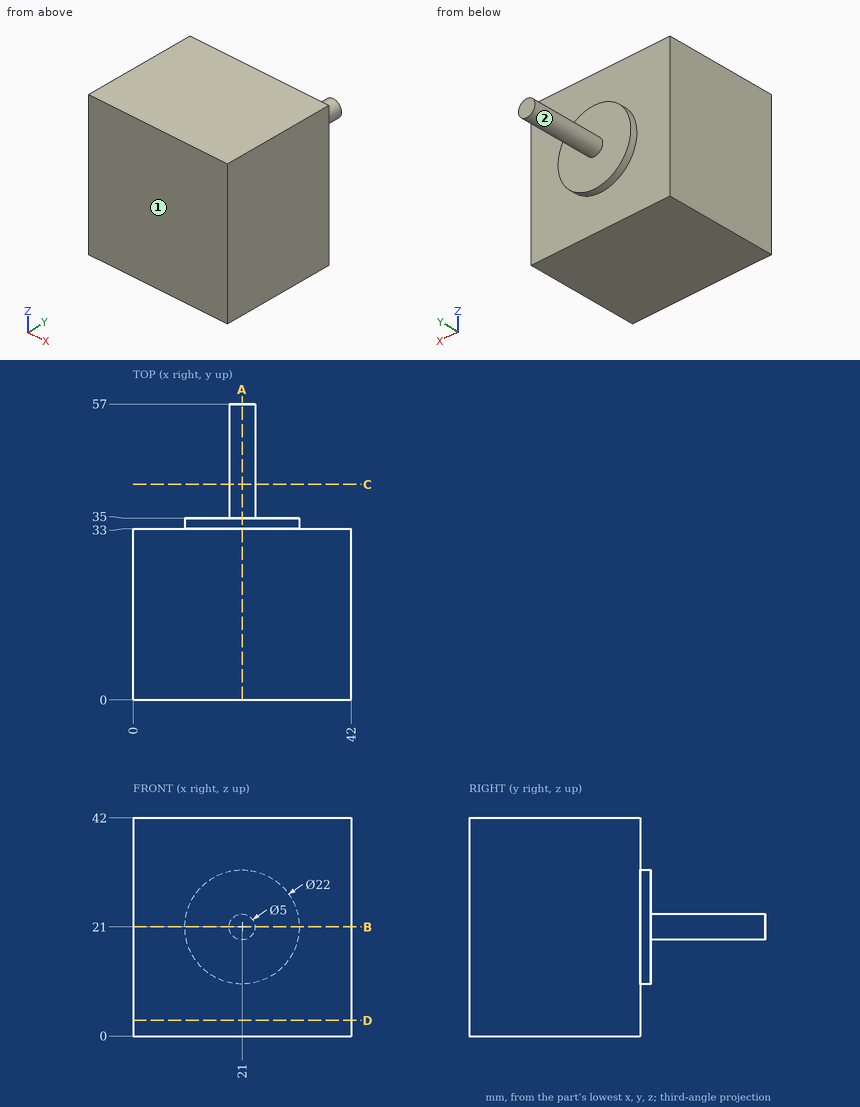
The figure shows three views and two pictorial views of one solid part (mm, origin at its lowest corner). Answer the questions. A direction names the side the tool comes from. Give positions to 0.01 mm unless a question says otherwise; leave off trailing zeros. Loops run counter-clockwise (first coordinate to the right, second up) from the corner with the lowest first, then second, coordinate; pieces in that order, holes last. Notation, with made-up numbers: (-19, 46) - (-3, 46) arc R32 cw to (-3, 76) - close; hole circle Ø4 at (-33, 83). An arc over 180 degrees is marked (long way). Use one line per item in the form item = value.
1. Find the intervals of material crossed by line 1 along Y through (x, z) = (21, 6); line 2 along Y through (x, z) = (22.5, 27); line 3 along X through (y, z) = (42, 19.5), in increasing order. Write a range as [from, to].
Calculated:
line_1 = [0, 33]
line_2 = [0, 35]
line_3 = [19, 23]
2. Section D-D on z = 3 is taken. Give the vertices of the cut face in (x, y).
Calculated:
outline = (0, 0) - (42, 0) - (42, 33) - (0, 33) - close
3. Section A-A on x = 21 is taken. Give the vertices of the cut face in (y, z).
Calculated:
outline = (0, 0) - (33, 0) - (33, 10) - (35, 10) - (35, 18.5) - (57, 18.5) - (57, 23.5) - (35, 23.5) - (35, 32) - (33, 32) - (33, 42) - (0, 42) - close
4. Section B-B on z = 21 is taken. Give the vertices of the cut face in (x, y), then the cut area to 3 significant figures.
Calculated:
outline = (0, 0) - (42, 0) - (42, 33) - (32, 33) - (32, 35) - (23.5, 35) - (23.5, 57) - (18.5, 57) - (18.5, 35) - (10, 35) - (10, 33) - (0, 33) - close
area = 1,540 mm^2
5. Section C-C on y = 41.5 is taken. Give the vertices of the cut face in (x, z), then the cut area to 3 significant figures.
Calculated:
outline = circle Ø5 at (21, 21)
area = 19.6 mm^2
6. Which of the six approach directions +Z, -Z, +X, -X, +Y, -Y give full straight-line access (tool end or side, diameter ignored) to the marked faces 1 and 2?
Calculated:
face_1 = +Z, -Z, +X, -X, -Y
face_2 = +Y
7. Given pin 1 Ø3 at (x, z) = (12.5, 25) entering from +Y; pin 2 Ø6 at (y, z) = (39.5, 19.5) entering from -X; pin 3 Ø1.5 at (y, z) = (36, 22.5) entering from -X, each flat-ended and moving along its own axis, determine where each tip first touches the part or whether it passes through.
Calculated:
pin_1 = 35
pin_2 = 18.5
pin_3 = 18.62
